Geometry check sheet. Reference: the model listing, model coordinates, mm. A direction names the side the tool comes from. Round coordinates to 2 decimals unless told otherwise and drop trailing zeros. Order: outer loops, then holes, each group sorted by start corner. A loop starts at its lowest first (then second) coordinate and runs counter-clockwise, first axis right, second up.
(1) Cross-section at D-D on y = 42. Enter the section's corners in (x, z).
(2) Cross-section at A-A on y = 5.65. Enter the section's corners in (x, z) (3 decimals).
(3) Cross-section at B-B on z = 4. Enter the section's corners in (x, y) (3 decimals), and give its area (3 significant figures).
(4) Gauge pin test, flat ends, axial feed: P1, Ø3, axis at x = 6.725, y = 5.65, coming from the +Z side; P2, Ø19, axis at x = 22.225, y = 21.36, coming from the +Z side; P3, Ø4, axis at x = 38.09, y = 12.34, coming from the -Z side. Record the tip position at first contact, or that the pin passes through.
(5) Cross-section at C-C on x = 38.5. Enter the section's corners in (y, z) (3 decimals), and give its area (3 significant figures).
(6) Set-up check for faces 5 (the face through (20.057, 11.598, 1.521)), 6 (the face through (42, 0, 23)), 7 (the face through (5.9, 32.43, 1.48)), 8 (the face through (36.455, 35.676, 42.971)), 9 (the face through (3, 27, 22)): record each of +Z, -Z, +X, -X, +Y, -Y from which the full face is reachable in a straight line by a thin tool's end or side.
(7) Thickness scan on L1, parallel to Z at x = 37, y = 10.5; L2, parallel to Z at x = 20, y = 32. Record the ranges inside material, lowest first.
(8) Draft check along Z on faces 1 (the face through (22, 34, 0)), 2 (the face through (22, 34, 44.45)), 3 (the face through (5.546, 6.731, 42.971)), 4 (the face through (22, 34, 3)). Enter one of: pulls with the +Z half, pulls with the -Z half, needs draft (parallel to the pull), parting line crosses it, or undercut.
from build123d import *

# Parameters (mm, degrees)
F0_W     = 44.45
F0_H     = 44.45
F0_W_2   = 38.45
F0_H_2   = 38.45
F1_DEPTH = 55.755
F2_R     = 10
F3_DEPTH = 44.451
F4_R     = 1.6
F4_R_2   = 12
F5_DEPTH = 5
F6_R     = 2.1
F7_DEPTH = 5


with BuildPart() as f1:
    # F0 (on Front) → F1 (new body)
    with BuildSketch(Plane.XZ):
        with Locations((22.225, 22.225)):
            Rectangle(F0_W, F0_H)
        with Locations((22.225, 22.225)):
            Rectangle(F0_W_2, F0_H_2, mode=Mode.SUBTRACT)
    extrude(amount=-F1_DEPTH)

    # F2 (on face) → F3 (cut, through all)
    with BuildSketch(Plane.XY.offset(44.45)):
        with Locations((22.225, 21.36)):
            Circle(F2_R)
    extrude(amount=-F3_DEPTH, mode=Mode.SUBTRACT)

    # F4 (on face) → F5 (cut)
    with BuildSketch(Plane.XY.offset(44.45)):
        with Locations((37.725, 5.65)):
            Circle(F4_R)
        with Locations((6.725, 5.65)):
            Circle(F4_R)
        with Locations((37.725, 36.65)):
            Circle(F4_R)
        with Locations((6.725, 36.65)):
            Circle(F4_R)
        with Locations((22.225, 21.36)):
            Circle(F4_R_2)
    extrude(amount=-F5_DEPTH, mode=Mode.SUBTRACT)

    # F6 (on face) → F7 (cut)
    with BuildSketch(Plane(origin=(0, 0, 0), x_dir=(1, 0, 0), z_dir=(0, 0, -1))):
        with Locations((38.090564, -12.340778)):
            Circle(F6_R)
        with Locations((6.359436, -30.379222)):
            Circle(F6_R)
    extrude(amount=-F7_DEPTH, mode=Mode.SUBTRACT)


solid = f1.part
Found:
1. outline: (0, 0) - (44.45, 0) - (44.45, 44.45) - (0, 44.45) - close; hole (3, 3) - (41.45, 3) - (41.45, 41.45) - (3, 41.45) - close
2. outline: (0, 0) - (44.45, 0) - (44.45, 44.45) - (39.325, 44.45) - (39.325, 41.45) - (41.45, 41.45) - (41.45, 3) - (3, 3) - (3, 41.45) - (5.125, 41.45) - (5.125, 44.45) - (0, 44.45) - close; (8.325, 41.45) - (36.125, 41.45) - (36.125, 44.45) - (8.325, 44.45) - close
3. outline: (0, 0) - (3, 0) - (3, 55.755) - (0, 55.755) - close; (41.45, 0) - (44.45, 0) - (44.45, 55.755) - (41.45, 55.755) - close
3. area: 335 mm2
4. P1: stops at z = 3
4. P2: passes through
4. P3: stops at z = 41.45
5. outline: (0, 0) - (10.281, 0) - (10.281, 3) - (0, 3) - close; (0, 41.45) - (4.25, 41.45) - (4.25, 44.45) - (0, 44.45) - close; (7.05, 41.45) - (35.25, 41.45) - (35.25, 44.45) - (7.05, 44.45) - close; (14.4, 0) - (55.755, 0) - (55.755, 3) - (14.4, 3) - close; (38.05, 41.45) - (55.755, 41.45) - (55.755, 44.45) - (38.05, 44.45) - close
5. area: 305 mm2
6. face 5: +Z, -Z
6. face 6: +Z, -Z, +X, -X, -Y
6. face 7: -Z
6. face 8: +Z
6. face 9: +Y, -Y
7. L1: z = 0 to 3, 41.45 to 44.45
7. L2: z = 0 to 3
8. face 1: pulls with the -Z half
8. face 2: pulls with the +Z half
8. face 3: needs draft
8. face 4: undercut
